from build123d import *

# Parameters (mm, degrees)
SKETCH1_W               = 294
SKETCH1_H               = 294
SKETCH1_W_2             = 228
SKETCH1_H_2             = 252
BOSS_EXTRUDE1_DEPTH     = 8
SKETCH2_R               = 8
CUT_EXTRUDE1_DEPTH      = 209.043264731
SKETCH4_R               = 8
CUT_EXTRUDE2_DEPTH      = 209.043264731
MIRROR3_COPY_1_SKETCH_R = 8
MIRROR3_COPY_1_DEPTH    = 209.043264731


with BuildPart() as part:
    # Sketch1 → Boss-Extrude1 (new body)
    with BuildSketch(Plane(origin=(0, 0, 0), x_dir=(1, 0, 0), z_dir=(0, 1, 0))):
        Rectangle(SKETCH1_W, SKETCH1_H)
        Rectangle(SKETCH1_W_2, SKETCH1_H_2, mode=Mode.SUBTRACT)
    extrude(amount=BOSS_EXTRUDE1_DEPTH)

    # Sketch2 → Cut-Extrude1 (cut, through all)
    with BuildSketch(Plane(origin=(0, 0, 0), x_dir=(1, 0, 0), z_dir=(0, 1, 0))):
        with Locations(Location((136, 136, 0), (0, 0, 270))):
            Circle(SKETCH2_R)
    cut_extrude1 = extrude(amount=CUT_EXTRUDE1_DEPTH, mode=Mode.SUBTRACT)

    # Mirror2: Cut-Extrude1 across plane
    add(cut_extrude1.mirror(Plane.XY), mode=Mode.SUBTRACT)

    # Sketch4 → Cut-Extrude2 (cut, through all)
    with BuildSketch(Plane(origin=(0, 8, 0), x_dir=(1, 0, 0), z_dir=(0, 1, 0))):
        with Locations((142.94, 0)):
            Circle(SKETCH4_R)
    cut_extrude2 = extrude(amount=-CUT_EXTRUDE2_DEPTH, mode=Mode.SUBTRACT)

    # Mirror3: Cut-Extrude1, Cut-Extrude2 across plane
    add(cut_extrude1.mirror(Plane(origin=(0, 0, 0), x_dir=(0, 0, 1), z_dir=(1, 0, 0))), mode=Mode.SUBTRACT)
    add(cut_extrude2.mirror(Plane(origin=(0, 0, 0), x_dir=(0, 0, 1), z_dir=(1, 0, 0))), mode=Mode.SUBTRACT)

    # Mirror3 copy 1 sketch → Mirror3 copy 1 (cut, through all)
    with BuildSketch(Plane(origin=(0, 0, 0), x_dir=(-1, 0, 0), z_dir=(0, 1, 0))):
        with Locations(Location((136, 136, 0), (0, 0, 270))):
            Circle(MIRROR3_COPY_1_SKETCH_R)
    extrude(amount=MIRROR3_COPY_1_DEPTH, mode=Mode.SUBTRACT)


solid = part.part
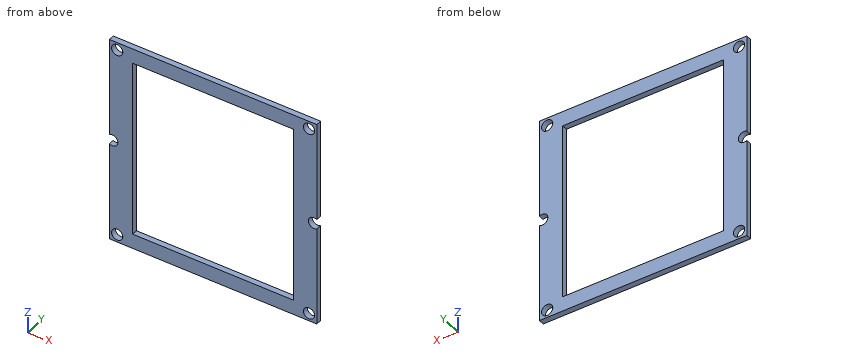
Can you work these out from the model? Positions are in its coordinate system, mm. Coordinates: 2 decimals unless noted, no trailing zeros. Write each loop counter-clockwise with the first axis right and the second up, starting at its lowest first coordinate (ties: lowest second). Pieces come first, ordered by that corner, then holes.
Q1. Imagine slicing it at B-B, the plane x = -19. List the corners of the cut face in (y, z) for me, plus the area to 3 significant figures.
Results found:
outline: (0, -147) - (8, -147) - (8, -126) - (0, -126) - close; (0, 126) - (8, 126) - (8, 147) - (0, 147) - close
area: 336 mm2
Q2. Please list where these lines run through material, in increasing order: L1, parallel to X at y = 3.5, z = 136; L2, parallel to X at y = 4.75, z = 39; L3, parallel to Z at x = 70.5, y = 3.5.
Results found:
L1: x = -147 to -144, -128 to 128, 144 to 147
L2: x = -147 to -114, 114 to 147
L3: z = -147 to -126, 126 to 147
Q3. Imagine slicing it at D-D, the plane z = 69.5. List the corners of the cut face in (x, y) for me, plus the area to 3 significant figures.
Results found:
outline: (-147, 0) - (-114, 0) - (-114, 8) - (-147, 8) - close; (114, 0) - (147, 0) - (147, 8) - (114, 8) - close
area: 528 mm2
Q4. Imagine slicing it at A-A, the plane z = 136. List the corners of the cut face in (x, y) for me, plus the area to 3 significant figures.
Results found:
outline: (-147, 0) - (-144, 0) - (-144, 8) - (-147, 8) - close; (-128, 0) - (128, 0) - (128, 8) - (-128, 8) - close; (144, 0) - (147, 0) - (147, 8) - (144, 8) - close
area: 2,100 mm2
Q5. Imagine slicing it at C-C, the plane y = 3.75. List the corners of the cut face in (x, z) for me.
Results found:
outline: (-147, -147) - (147, -147) - (147, -6.89) arc R8 cw (long way) to (147, 6.89) - (147, 147) - (-147, 147) - (-147, 6.89) arc R8 cw (long way) to (-147, -6.89) - close; hole circle Ø16 at (-136, -136); hole circle Ø16 at (-136, 136); hole (-114, -126) - (114, -126) - (114, 126) - (-114, 126) - close; hole circle Ø16 at (136, -136); hole circle Ø16 at (136, 136)
Q6. For P1, Ø9.5, axis at x = 136, z = -136, coming from the -Y side; P2, Ø18.5, axis at x = 136, z = 136, coming from the -Y side, each with a flat end and sliding along its axis, tell me the tip position at first contact or that it passes through.
Results found:
P1: passes through
P2: stops at y = 0
